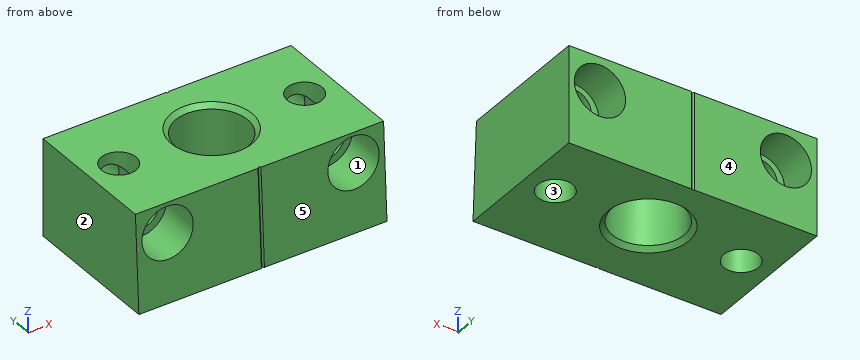
```python
from build123d import *

# Parameters (mm, degrees)
SKETCH1_W          = 64.008
SKETCH1_H          = 36.4998
SKETCH1_R          = 9.2585
SKETCH1_R_2        = 4.4958
EXTRUDE1_DEPTH     = 24.9936
CUT_EXTRUDE1_DEPTH = 65.008
LPATTERN1_COUNT    = 2
LPATTERN1_PITCH    = 47.9552
CHAMFER1_SIZE      = 1.1555
CUT_EXTRUDE2_DEPTH = 25.9936001
CUT_EXTRUDE3_DEPTH = 27.869599175


with BuildPart() as part:
    # Sketch1 → Extrude1 (new body)
    with BuildSketch(Plane.XY):
        with Locations((0, -1.2573)):
            Rectangle(SKETCH1_W, SKETCH1_H)
        Circle(SKETCH1_R, mode=Mode.SUBTRACT)
        with Locations((-23.9776, 0)):
            Circle(SKETCH1_R_2, mode=Mode.SUBTRACT)
        with Locations((23.9776, 0)):
            Circle(SKETCH1_R_2, mode=Mode.SUBTRACT)
    extrude(amount=EXTRUDE1_DEPTH)

    # Sketch2 → Cut-Extrude1 (cut, through all)
    with BuildSketch(Plane(origin=(32.004, 0, 0), x_dir=(0, 0, -1), z_dir=(1, 0, 0))):
        Polygon((0, -19.5072), (-24.9936, -18.197340928), (-24.9936, -19.5072), align=None)
    extrude(amount=-CUT_EXTRUDE1_DEPTH, mode=Mode.SUBTRACT)

    # Sketch3 → Cut-Revolve1 (revolve, cut)
    with BuildSketch(Plane(origin=(-23.9776, 0, 0), x_dir=(0, 0, -1), z_dir=(1, 0, 0)), mode=Mode.PRIVATE) as cut_revolve1_sk:
        Polygon((-10.8966, -18.936133392), (-10.8966, -8.4074), (-12.827, -8.4074), (-12.827, 16.9926), (-17.5006, 16.9926), (-17.5006, -18.936133392), align=None)
    cut_revolve1 = revolve(cut_revolve1_sk.sketch.rotate(Axis((-23.9776, 16.931830478, 17.5006), (0, -1, 0)), 180), axis=Axis((-23.9776, 16.931830478, 17.5006), (0, -1, 0)), mode=Mode.SUBTRACT)  # turned: the seam where the file's is

    # Sketch4 → Cut-Revolve2 (revolve, cut)
    with BuildSketch(Plane(origin=(-23.9776, 0, 0), x_dir=(0, 0, -1), z_dir=(1, 0, 0)), mode=Mode.PRIVATE) as cut_revolve2_sk:
        Polygon((-9.761726171, 16.9926), (-10.313289005, 6.468154162), (-16.908238453, 6.813780817), (-16.356675618, 17.338226655), align=None)
    cut_revolve2 = revolve(cut_revolve2_sk.sketch.rotate(Axis((-23.9776, 21.413064128, 16.143122435), (0, -0.998629535, 0.052335956)), 180), axis=Axis((-23.9776, 21.413064128, 16.143122435), (0, -0.998629535, 0.052335956)), mode=Mode.SUBTRACT)  # turned: the seam where the file's is

    # LPattern1: Cut-Revolve1, Cut-Revolve2 ×2
    with Locations(*[(i * LPATTERN1_PITCH, 0, 0) for i in range(1, LPATTERN1_COUNT)]):
        add(cut_revolve1, mode=Mode.SUBTRACT)
        add(cut_revolve2, mode=Mode.SUBTRACT)

    # Chamfer1
    chamfer1_edges = [part.edges().sort_by_distance(p)[0] for p in [
        (-9.2585, 0, 0),
        (-9.2585, 0, 24.9936),
    ]]
    chamfer(chamfer1_edges, length=CHAMFER1_SIZE)

    # Sketch5 → Cut-Extrude2 (cut, through all)
    with BuildSketch(Plane(origin=(0, 0, 0), x_dir=(-1, 0, 0), z_dir=(0, 0, -1))):
        Polygon((-0.381, 16.9926), (0, 16.6116), (0.381, 16.9926), align=None)
    extrude(amount=-CUT_EXTRUDE2_DEPTH, mode=Mode.SUBTRACT)

    # Sketch6 → Cut-Extrude3 (cut, through all)
    with BuildSketch(Plane(origin=(0, -0.053431241, -1.019528819), x_dir=(-1, 0, 0), z_dir=(0, -0.052335956, -0.998629535))):
        Polygon((0.381, -19.48046606), (0, -19.09946606), (-0.381, -19.48046606), align=None)
    extrude(amount=-CUT_EXTRUDE3_DEPTH, mode=Mode.SUBTRACT)


solid = part.part
```
CAD build for the part. Positions are in the model's coordinates, mm. Face numbers are marked on the shaded views. A direction names the side the tool comes from. Give positions to 0.01 mm unless a question says otherwise; leave off trailing zeros. Order: outer loops, then holes, each group sorted by start corner. A loop starts at its lowest first (then second) coordinate and runs counter-clockwise, first axis right, second up.
(1) Saw through at B-B, the plane x = -20.5. Give the cut face in (y, z), then the cut area to 3 significant figures.
(2) Saw through at A-A, the plane y = 0. Give the cut face in (x, z).
(3) Flat gauge pins, fed straight in: pin 1 (8.5 mm diameter, centred on x = -23.98, z = 17.5, fed in from -Y); pin 2 (6 mm diameter, centred on x = -2.5, z = 6, fed in from -Y); pin 3 (1 mm diameter, centred on x = -2, z = 6, fed in from -Y); pin 4 (1.5 mm diameter, centred on x = -5.5, z = 13.5, fed in from -Y). Where does each tip first touch, or does it go through?
(4) Saw through at C-C, the plane z = 19.75. State how many separate pieces and enclosed holes the cut face has, then the cut area to 3 significant figures.
(5) Tool access for the marked faces 1 and 2: list every direction of +Z, -Z, +X, -X, +Y, -Y with a clear straight run to the whole face (end or side of a thin tool).
(6) Drill centre lines: L1, parallel to Y at x = -24, z = 22.25; L2, parallel to X at y = 12, z = 12.25; L3, parallel to X at y = 9.5, z = 16.5. Where is each one in solid material? Low to high.
(7) Mould opens along Y. For the marked faces 3, 4 and 5 say: released by +Y, released by -Y, zero draft, split by the parting line, or undercut.
(8) Saw through at D-D, the plane z = 7. Give the cut face in (x, y), then the cut area to 3 significant figures.
Results found:
1. outline: (-19.51, 0) - (-2.85, 0) - (-2.85, 14.38) - (-8.41, 14.38) - (-8.41, 11.89) - (-18.88, 11.89) - close; (-18.3, 23.11) - (-8.41, 23.11) - (-8.41, 20.62) - (-2.85, 20.62) - (-2.85, 24.99) - (-18.2, 24.99) - close; (2.85, 0) - (16.99, 0) - (16.99, 10.75) - (6.52, 11.3) - (6.68, 14.38) - (2.85, 14.38) - close; (2.85, 20.62) - (7.01, 20.62) - (7.11, 22.51) - (16.99, 22) - (16.99, 24.99) - (2.85, 24.99) - close
1. area: 465 mm2
2. outline: (-32, 0) - (-28.47, 0) - (-28.47, 16.22) arc R4.67 cw to (-28.47, 18.78) - (-28.47, 24.99) - (-32, 24.99) - close; (-19.48, 0) - (-10.41, 0) - (-9.26, 1.16) - (-9.26, 23.84) - (-10.41, 24.99) - (-19.48, 24.99) - (-19.48, 18.78) arc R4.67 cw to (-19.48, 16.22) - close; (9.26, 1.16) - (10.41, 0) - (19.48, 0) - (19.48, 16.22) arc R4.67 cw to (19.48, 18.78) - (19.48, 24.99) - (10.41, 24.99) - (9.26, 23.84) - close; (28.47, 0) - (32, 0) - (32, 24.99) - (28.47, 24.99) - (28.47, 18.78) arc R4.67 cw to (28.47, 16.22) - close
3. pin 1: passes through
3. pin 2: stops at y = -19.35
3. pin 3: stops at y = -19.22
3. pin 4: stops at y = -18.84
4. separate pieces: 3
4. enclosed holes: 1
4. area: 1,260 mm2
5. face 1: -Y
5. face 2: +Z, -Z, -X, +Y, -Y
6. L1: y = -8.41 to -4.5, 4.5 to 7.09
6. L2: x = -32 to -28.92, -19.04 to 19.04, 28.92 to 32
6. L3: x = -32 to -30.58, -17.38 to 17.38, 30.58 to 32
7. face 3: undercut
7. face 4: released by +Y
7. face 5: released by -Y
8. outline: (-32, -19.14) - (-0.38, -19.14) - (0, -18.76) - (0.38, -19.14) - (32, -19.14) - (32, 16.99) - (0.38, 16.99) - (0, 16.61) - (-0.38, 16.99) - (-32, 16.99) - close; hole circle Ø8.99 at (-23.98, 0); hole circle Ø18.52 at (0, 0); hole circle Ø8.99 at (23.98, 0)
8. area: 1,920 mm2
